Model file for the job. Use its own axes, mm. Face numbers are marked on the shaded views. Round coordinates to 2 decimals unless told otherwise and drop trailing zeros. Loops run counter-clockwise (first coordinate to the right, second up) from the corner with the lowest first, then second, coordinate; pieces in that order, holes last. Notation, with made-up numbers: M -18,32.5 L 21,32.5 A30 cw 21,57.5 Z; hole C 50.25,-34 d2. An arc over 180 degrees is marked long. Use a Markdown table: item, result. Add a question column.
Item 1: Saw through at D-D on z = -38. Write the cut outline in (x, y).
Item 2: Saw through at C-C on y = 26. Write the cut outline in (x, z), then the cut area to 3 significant figures.
Item 3: Two-plate mould, pull along X, no slides. Class the marked faces 1, 2, 3 and 4: +X half, -X half, draft (parallel to the pull), parting line (faces both ways), or undercut.
Item 4: Saw through at B-B on x = 65.5. Write the cut outline in (y, z), then the cut area to 3 significant figures.
Item 5: Saw through at A-A on z = -50. Write the cut outline in (x, y).
Item 6: Wall check: L1, parallel to X at y = 41, z = -3.5; L2, parallel to Y at x = 73.45, z = -50; L3, parallel to Z at x = 47.5, y = 9.5. Give the ranges that are in metal, low to high. Write a range as from..to.
Item 7: Pin check, flat tips, straight feed: P1, Ø4, axis at y = 39.5, z = 3, coming from the +X side; P2, Ø1.8, axis at x = 17.5, z = -40.5, coming from the +Y side; P3, Ø1.8, axis at x = 18, z = -16.5, coming from the -Y side; P4, Ø3, axis at y = 36.59, z = -50, coming from the +X side. Stop position of each tip, or through.
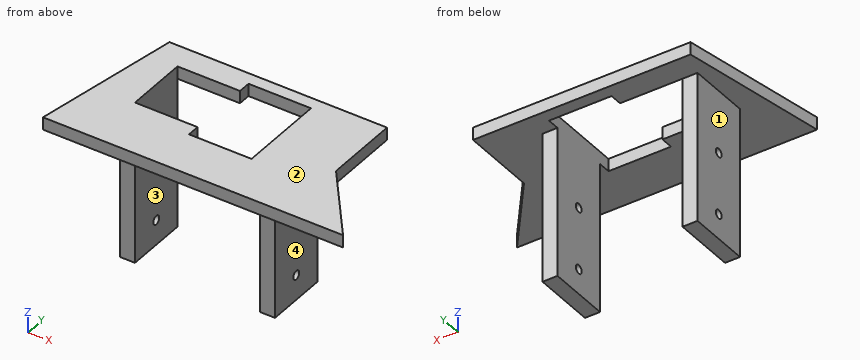
Autodesk Inventor part; units mm, degrees
ref_plane "YZ Plane" through (0, 0, 0) normal (1, 0, 0) x (0, 1, 0)
ref_plane "XZ Plane" through (0, 0, 0) normal (0, 1, 0) x (-1, 0, 0)
ref_plane "XY Plane" through (0, 0, 0) normal (0, 0, 1) x (1, 0, 0)
sketch "Szkic1" plane through (0, 0, 0) normal (0, 0, 1) x (1, 0, 0)
  line L0 (0, 0) -> (120, 0)
  line L1 (0, 0) -> (10.4189, 59.0885)
  line L2 (0, 0) -> (60, 0) construction
  line L3 (10.4189, 59.0885) -> (70.4189, 59.0885)
  line L4 (70.4189, 59.0885) -> (97.4189, 59.0885)
  line L5 (97.4189, 59.0885) -> (97.4189, 29.0885)
  line L6 (97.4189, 29.0885) -> (120, 0)
  line L7 (20.4189, 49.0885) -> (70.4189, 49.0885)
  line L8 (70.4189, 49.0885) -> (70.4189, 24.0885)
  line L9 (70.4189, 24.0885) -> (20.4189, 24.0885)
  line L10 (20.4189, 24.0885) -> (20.4189, 49.0885)
  dimension "d0" = 120
  dimension "d1" = 60
  dimension "d2" = 80
  dimension "d3" = 60
  dimension "d4" = 27
  dimension "d5" = 30
  dimension "d6" = 50
  dimension "d7" = 25
  dimension "d8" = 10
  dimension "d9" = 10
extrude "Wyciągnięcie proste1" add sketch "Szkic1" along normal blind 5
sketch "Szkic2" plane through (0, 0, 0) normal (0, 0, -1) x (-1, 0, 0)
  line L0 (-20.4189, 24.0885) -> (-20.4189, 49.0885)
  line L1 (-20.4189, 49.0885) -> (-14.4189, 49.0885)
  line L2 (-14.4189, 49.0885) -> (-14.4189, 24.0885)
  line L3 (-14.4189, 24.0885) -> (-20.4189, 24.0885)
  line L4 (-20.4189, 24.0885) -> (-20.4189, 49.0885)
  point P0 (0, 0)
  dimension "d12" = 6
extrude "Wyciągnięcie proste2" add sketch "Szkic2" along normal blind 30
sketch "Szkic3" plane through (0, 0, -30) normal (0, 0, -1) x (-1, 0, 0)
  line L0 (-20.4189, 24.0885) -> (-20.4189, 49.0885)
  line L1 (-20.4189, 24.0885) -> (-14.4189, 24.0885)
  line L2 (-20.4189, 49.0885) -> (-14.4189, 49.0885)
  line L3 (-14.4189, 49.0885) -> (-14.4189, 24.0885)
  line L4 (-14.4189, 24.0885) -> (-20.4189, 24.0885)
  line L5 (-20.4189, 24.0885) -> (-20.4189, 49.0885)
  point P0 (0, 0)
extrude "Wyciągnięcie proste3" add sketch "Szkic3" along normal blind 30
sketch "Szkic4" plane through (0, 0, 0) normal (0, 0, -1) x (-1, 0, 0)
  line L0 (-70.4189, 49.0885) -> (-70.4189, 24.0885)
  line L1 (-70.4189, 49.0885) -> (-76.4189, 49.0885)
  line L2 (-76.4189, 49.0885) -> (-76.4189, 24.0885)
  line L3 (-76.4189, 24.0885) -> (-70.4189, 24.0885)
  line L4 (-70.4189, 24.0885) -> (-70.4189, 49.0885)
  point P0 (0, 0)
  dimension "d17" = 6
extrude "Wyciągnięcie proste4" add sketch "Szkic4" along normal up to surface (60 mm away)
sketch "Szkic5" plane through (14.4189, 24.0885, 0) normal (-1, 0, 0) x (0, 0, 1)
  line L0 (-60, 0) -> (-60, 25)
  point P0 (0, -24.0885)
  point P1 (-50, 12.5)
  point P2 (-60, 12.5)
  dimension "d20" = 10
hole "Otwór1" at (14.4189, 36.5885, -50) direction (1, 0, 0) diameter 3.5 depth 6
sketch "Szkic7" plane through (76.4189, 24.0885, 0) normal (1, 0, 0) x (0, 0, -1)
  circle A0 centre (50, 12.5) radius 1.75
  point P0 (0, -24.0885)
hole "Otwór2" at (76.4189, 36.5885, -50) direction (-1, 0, 0) diameter 3.5 depth 6
sketch "Szkic8" plane through (14.4189, 24.0885, 0) normal (-1, 0, 0) x (0, 0, 1)
  point P0 (0, -24.0885)
  point P1 (-25.1365, 12.5)
hole "Otwór3" at (14.4189, 36.5885, -25.1365) direction (1, 0, 0) diameter 3.4 end through all
sketch "Szkic10" plane through (0, 0, 0) normal (0, 0, -1) x (-1, 0, 0)
  line L0 (-70.4189, 49.0885) -> (-70.4189, 24.0885)
  line L1 (-70.4189, 49.0885) -> (-70.4189, 54.0885)
  line L2 (-70.4189, 54.0885) -> (-45.4189, 54.0885)
  line L3 (-70.4189, 24.0885) -> (-70.4189, 19.0885)
  line L4 (-70.4189, 19.0885) -> (-45.4189, 19.0885)
  line L5 (-45.4189, 19.0885) -> (-45.4189, 54.0885)
  point P0 (0, 0)
  dimension "d49" = 5
  dimension "d50" = 5
extrude "Wyciągnięcie proste7" cut sketch "Szkic10" against normal blind 10
properties part number "podstawa"
Entries:
| question | item | result |
|---|---|---|
| 1 | outline | M 14.42,24.09 L 20.42,24.09 L 20.42,49.09 L 14.42,49.09 Z; M 70.42,24.09 L 76.42,24.09 L 76.42,49.09 L 70.42,49.09 Z |
| 2 | outline | M 4.58,0 L 14.42,0 L 14.42,-60 L 20.42,-60 L 20.42,5 L 4.58,5 Z; M 70.42,-60 L 76.42,-60 L 76.42,0 L 99.82,0 L 99.82,5 L 70.42,5 Z |
| 2 | area | 946 mm2 |
| 3 | face 1 | -X half |
| 3 | face 2 | draft |
| 3 | face 3 | undercut |
| 3 | face 4 | +X half |
| 4 | outline | M 0,0 L 19.09,0 L 19.09,5 L 0,5 Z; M 54.09,0 L 59.09,0 L 59.09,5 L 54.09,5 Z |
| 4 | area | 120 mm2 |
| 5 | outline | M 14.42,24.09 L 20.42,24.09 L 20.42,34.84 L 14.42,34.84 Z; M 14.42,38.34 L 20.42,38.34 L 20.42,49.09 L 14.42,49.09 Z; M 70.42,24.09 L 76.42,24.09 L 76.42,34.84 L 70.42,34.84 Z; M 70.42,38.34 L 76.42,38.34 L 76.42,49.09 L 70.42,49.09 Z |
| 6 | L1 | 14.42..20.42, 70.42..76.42 |
| 6 | L2 | 24.09..34.84, 38.34..49.09 |
| 6 | L3 | 0..5 |
| 7 | P1 | x = 97.42 |
| 7 | P2 | y = 49.09 |
| 7 | P3 | y = 24.09 |
| 7 | P4 | through |
